Here's how the part is built. I have some questions about the finished solid (model axes, mm). A direction names the side the tool comes from. Round coordinates to 2 decimals unless told otherwise and drop trailing zeros. Write each loop counter-clockwise with the first axis right and the second up, starting at its lowest first coordinate (ties: lowest second). Pieces come first, ordered by that corner, then holes. Notation, with made-up numbers: (21.25, 70) -> (28.25, 70) arc R10 ccw to (28.25, 85) -> close; hole circle Ø7 at (71.5, 12). An arc over 180 degrees is marked (long way). Answer as CSV lines item,"result".
from build123d import *

# Parameters (mm, degrees)
BASE_FLANGE2_START           = -3
BASE_FLANGE2_OUTLINE_R       = 10
BASE_FLANGE2_DEPTH           = 3
EDGE_FLANGE1_STRIP_W         = 13.4732
EDGE_FLANGE1_STRIP_H         = 3
EDGE_FLANGE1_STRIP_CUT_DEPTH = 10
EDGE_FLANGE1_DEPTH           = 10
BOSS_EXTRUDE1_START          = -3.5
BOSS_EXTRUDE1_DEPTH          = 3
TAP_DRILL_FOR_M5X0_8_TAP2_D  = 4.2
CIRPATTERN2_COUNT            = 6


# Read off the part's stored shape, not the designer's step: Base-Flange2
# Sheet-metal steps are written as plain solids
with BuildPart() as part:
    # Base-Flange2 outline → Base-Flange2 (new body)
    with BuildSketch(Plane.XY.offset(BASE_FLANGE2_START)):
        with BuildLine():
            Line((5, 70), (-5, 70))
            Line((-5, 70), (-5, 24.494897428))
            ThreePointArc((-5, 24.494897428), (0, -25), (5, 24.494897428))
            Line((5, 24.494897428), (5, 70))
        make_face()
        Circle(BASE_FLANGE2_OUTLINE_R, mode=Mode.SUBTRACT)
    extrude(amount=BASE_FLANGE2_DEPTH)

    # Edge-Flange1 strip (across the edge) → Edge-Flange1 strip cut (cut)
    with BuildSketch(Plane(origin=(5, 70, 0), x_dir=(0, -1, 0), z_dir=(-1, 0, 0))):
        with Locations((-6, -1.5)):
            Rectangle(EDGE_FLANGE1_STRIP_W, EDGE_FLANGE1_STRIP_H)
    extrude(amount=EDGE_FLANGE1_STRIP_CUT_DEPTH, mode=Mode.SUBTRACT)

    # Edge-Flange1 section (across the edge) → Edge-Flange1 (add)
    with BuildSketch(Plane(origin=(5, 70, 0), x_dir=(0, -1, 0), z_dir=(-1, 0, 0))):
        with BuildLine():
            Line((-3, 0.7366), (-3, 50))
            Line((-3, 50), (0, 50))
            Line((0, 50), (0, 0.7366))
            ThreePointArc((0, 0.7366), (0.215745145, 0.215745145), (0.7366, 0))
            Line((0.7366, 0), (0.7366, -3))
            ThreePointArc((0.7366, -3), (-1.905575199, -1.905575199), (-3, 0.7366))
        make_face()
    extrude(amount=EDGE_FLANGE1_DEPTH)

    # Sketch13 → Boss-Extrude1 (add)
    with BuildSketch(Plane(origin=(5, 0, 0), x_dir=(0, 0, -1), z_dir=(1, 0, 0)).offset(BOSS_EXTRUDE1_START)):
        with BuildLine():
            Line((-50, 70), (-0.74, 70))
            ThreePointArc((-0.74, 70), (-0.216740982, 69.783259018), (0, 69.26))
            Line((0, 69.26), (0, 10))
            Line((0, 10), (-50, 70))
        make_face()
    extrude(amount=-BOSS_EXTRUDE1_DEPTH)

    # Tap Drill for M5x0.8 Tap2 (through all)
    with Locations(Plane.XY):
        with Locations((17.5, 0)):
            tap_drill_for_m5x0_8_tap2 = Hole(TAP_DRILL_FOR_M5X0_8_TAP2_D / 2)

    # CirPattern2: Tap Drill for M5x0.8 Tap2 ×6 about axis
    cirpattern2_axis = Axis((0, 0, 0), (0, 0, 1))
    for i in range(1, CIRPATTERN2_COUNT):
        add(tap_drill_for_m5x0_8_tap2.rotate(cirpattern2_axis, i * 360 / CIRPATTERN2_COUNT), mode=Mode.SUBTRACT)


solid = part.part
Item 1: Will these pins go through, and if not, where does the flat tip stop? pin 1 (14.5 mm diameter, centred on y = 55, z = 34, fed in from +X); pin 2 (11 mm diameter, centred on x = 0.5, z = 21.5, fed in from -Y); pin 3 (15 mm diameter, centred on y = 33, z = 20.5, fed in from -X).
Results found:
pin 1,"stops at x = 1.5"
pin 2,"stops at y = 29.2"
pin 3,"stops at x = -1.5"
Item 2: Suppose I cut it at A-A, the plane y = 0. List the corners of the cut face in (x, z) for me.
Results found:
outline,"(-25, -3) -> (-19.6, -3) -> (-19.6, 0) -> (-25, 0) -> close; (-15.4, -3) -> (-10, -3) -> (-10, 0) -> (-15.4, 0) -> close; (10, -3) -> (15.4, -3) -> (15.4, 0) -> (10, 0) -> close; (19.6, -3) -> (25, -3) -> (25, 0) -> (19.6, 0) -> close"
Item 3: I need wall thicknesses on L1, parallel to Y at x = -8.75, z = -0.75; L2, parallel to Z at x = 3, y = 15.5; L3, parallel to X at y = 63.5, z = 44. Which ranges of each line are inside material? Lowest first, please.
Results found:
L1,"y = -23.42 to -17.26, -13.06 to -4.84, 4.84 to 13.06, 17.26 to 23.42"
L2,"z = -3 to 0"
L3,"x = -1.5 to 1.5"
Item 4: Suppose I cut it at B-B, the plane x = -8.75. List the corners of the cut face in (y, z) for me, then the cut area to 3 significant figures.
Results found:
outline,"(-23.42, -3) -> (-17.26, -3) -> (-17.26, 0) -> (-23.42, 0) -> close; (-13.06, -3) -> (-4.84, -3) -> (-4.84, 0) -> (-13.06, 0) -> close; (4.84, -3) -> (13.06, -3) -> (13.06, 0) -> (4.84, 0) -> close; (17.26, -3) -> (23.42, -3) -> (23.42, 0) -> (17.26, 0) -> close"
area,"86.3 mm²"
Item 5: For faces 4 (the flat face through (2, 70, 26)), 5 (the flat face through (1.5, 47, 19)), 6 (the flat face through (0, 72, 50)), 7 (the flat face through (-1.5, 47, 19)), 8 (the flat face through (-5, 70.2, 15.8)), which set-ups out of +Z, -Z, +X, -X, +Y, -Y let a thin tool reach every point of the face, with its end or its side?
Results found:
face 4,"+Z, -Y"
face 5,"+Z, +X, -Y"
face 6,"+Z, +X, -X, +Y, -Y"
face 7,"+Z, -X, -Y"
face 8,"+Z, -Z, -X, +Y"
Item 6: Suppose I cut it at D-D, the plane x = -17. List the corners of the cut face in (y, z) for me, then the cut area to 3 significant figures.
Results found:
outline,"(-18.33, -3) -> (-2.04, -3) -> (-2.04, 0) -> (-18.33, 0) -> close; (2.04, -3) -> (18.33, -3) -> (18.33, 0) -> (2.04, 0) -> close"
area,"97.7 mm²"
Item 7: If we mould it in two halves opening along X, with no side actions, what happens to faces 1 (the flat face through (-2, 12, 0)), 2 (the cylindrical face through (9.879, -16.926, -1.521)), 3 (the flat face through (5, 70.2, 15.8))? For each: pulls with the +X half, pulls with the -X half, needs draft (parallel to the pull), parting line crosses it, or undercut.
Results found:
face 1,"needs draft"
face 2,"undercut"
face 3,"pulls with the +X half"
Item 8: Suppose I cut it at C-C, the plane z = 33.5. List the corners of the cut face in (x, y) for me, then the cut area to 3 significant figures.
Results found:
outline,"(-5, 70) -> (-1.5, 70) -> (-1.5, 50.2) -> (1.5, 50.2) -> (1.5, 70) -> (5, 70) -> (5, 73) -> (-5, 73) -> close"
area,"89.4 mm²"
